Part model, mm, in its own coordinate system. Face numbers are marked on the shaded views. A direction names the side the tool comes from. Round coordinates to 2 decimals unless told otherwise and drop trailing zeros. Loops run counter-clockwise (first coordinate to the right, second up) from the corner with the lowest first, then second, coordinate; pieces in that order, holes last.
(1) Tool access for the marked faces 1 and 2: list every direction of +Z, -Z, +X, -X, +Y, -Y with a clear straight run to the whole face (end or side of a thin tool).
(2) Cut at A-A on y = -1.1. List the corners of the cut face in (x, z), then the cut area to 3 significant figures.
(3) Cut at D-D on z = 6.5. List the corners of the cut face in (x, y), then the cut area to 3 significant figures.
(4) Probe probe 1 along Z at (x, y) = (0, -14.45); probe 2 along Z at (x, y) = (0, -14.6); probe 3 along Y at (x, z) = (0.5, 2.5). List the from-to ranges inside material, lowest first.
(5) Cut at C-C on x = -4. List the corners of the cut face in (y, z).
(6) Mould opens along Z. For the marked faces 3, 4, 5 and 6 say: +Z half, -Z half, draft (parallel to the pull), parting line (faces both ways), or undercut.
(7) Flat gauge pins, fed straight in: pin 1 (8 mm diameter, centred on x = -3.5, y = 13.5, fed in from +Z); pin 2 (3.5 mm diameter, centred on x = 0, y = 16.2, fed in from +Z); pin 3 (6 mm diameter, centred on x = 2, z = 21.5, fed in from +Y). Where does each tip first touch, or does it go through?
(8) Cut at B-B on x = 0. List the corners of the cut face in (y, z).
from build123d import *

# Parameters (mm, degrees)
SKETCH1_R           = 2.25
BOSS_EXTRUDE1_DEPTH = 3
CIRPATTERN1_COUNT   = 2
CIRPATTERN1_ANGLE   = 90
FILLET1_R           = 3


with BuildPart() as part:
    # Sketch1 → Boss-Extrude1 (new body)
    with BuildSketch(Plane.XY):
        with BuildLine():
            Line((-8.4, 15.8), (-8.4, -15.8))
            Line((-8.4, -15.8), (8.4, -15.8))
            Line((8.4, -15.8), (8.4, 15.8))
            ThreePointArc((8.4, 15.8), (0, 24.2), (-8.4, 15.8))
        make_face()
        with Locations((0, 16.2)):
            Circle(SKETCH1_R, mode=Mode.SUBTRACT)
        with Locations((0, -1.1)):
            Circle(SKETCH1_R, mode=Mode.SUBTRACT)
    boss_extrude1 = extrude(amount=BOSS_EXTRUDE1_DEPTH)

    # CirPattern1: Boss-Extrude1 ×2 about axis
    cirpattern1_axis = Axis((-9.24, -14.3, 1.5), (1, 0, 0))
    for i in range(1, CIRPATTERN1_COUNT):
        add(boss_extrude1.rotate(cirpattern1_axis, i * CIRPATTERN1_ANGLE / (CIRPATTERN1_COUNT - 1)))

    # Fillet1
    fillet1_edges = [part.edges().sort_by_distance(p)[0] for p in [
        (0, -15.8, 0),
    ]]
    fillet(fillet1_edges, radius=FILLET1_R)


solid = part.part
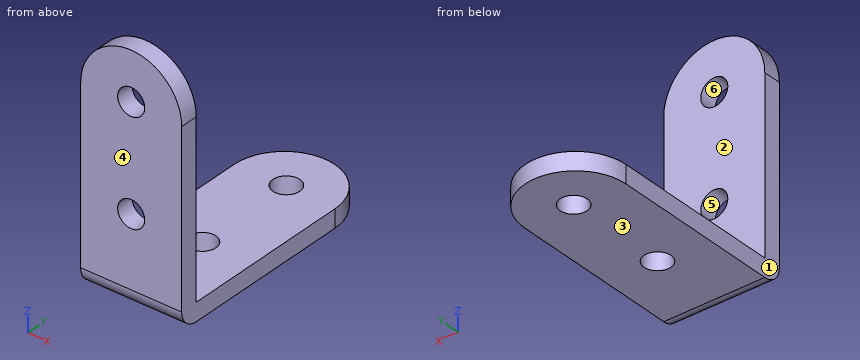
Final values:
1. face 1: +Z, -Z, -X, +Y, -Y
1. face 2: +Z, +X, -X, +Y
2. outline: (-8.4, 0) - (-2.25, 0) - (-2.25, 3) - (-8.4, 3) - close; (2.25, 0) - (8.4, 0) - (8.4, 3) - (2.25, 3) - close
2. area: 36.9 mm2
3. outline: (-8.4, -15.8) - (8.4, -15.8) - (8.4, -12.8) - (-8.4, -12.8) - close
3. area: 50.4 mm2
4. probe 1: z = 0.49 to 12.45, 16.95 to 29.75, 34.25 to 40
4. probe 2: z = 0.6 to 12.45, 16.95 to 29.75, 34.25 to 40
4. probe 3: y = -15.76 to -3.29, 1.09 to 14.01, 18.39 to 24.19
5. outline: (-15.8, 3) arc R3 ccw to (-12.8, 0) - (23.19, 0) - (23.19, 3) - (-12.8, 3) - (-12.8, 38.99) - (-15.8, 38.99) - close
6. face 3: -Z half
6. face 4: draft
6. face 5: undercut
6. face 6: undercut
7. pin 1: stops at z = 3
7. pin 2: passes through
7. pin 3: stops at y = -12.8
8. outline: (-15.8, 3) arc R3 ccw to (-12.8, 0) - (-3.35, 0) - (-3.35, 3) - (-12.8, 3) - (-12.8, 12.45) - (-15.8, 12.45) - close; (-15.8, 16.95) - (-12.8, 16.95) - (-12.8, 29.75) - (-15.8, 29.75) - close; (-15.8, 34.25) - (-12.8, 34.25) - (-12.8, 40) - (-15.8, 40) - close; (1.15, 0) - (13.95, 0) - (13.95, 3) - (1.15, 3) - close; (18.45, 0) - (24.2, 0) - (24.2, 3) - (18.45, 3) - close
